from build123d import *

# Parameters (mm, degrees)
BOSS_EXTRUDE2_DEPTH = 20
SKETCH3_R           = 30
SKETCH3_R_2         = 15
BOSS_EXTRUDE3_DEPTH = 30
SKETCH5_R           = 15
BOSS_EXTRUDE4_DEPTH = 70
FILLET1_R           = 5


with BuildPart() as part:
    # Sketch1 → Boss-Extrude2 (new body)
    with BuildSketch(Plane(origin=(0, 0, 0), x_dir=(1, 0, 0), z_dir=(0, 1, 0))):
        with BuildLine():
            Line((-121.213203436, 21.213203436), (-21.213203436, 121.213203436))
            ThreePointArc((-21.213203436, 121.213203436), (0, 70), (21.213203436, 121.213203436))
            Line((21.213203436, 121.213203436), (121.213203436, 21.213203436))
            ThreePointArc((121.213203436, 21.213203436), (72.283614025, 11.480502971), (100, -30))
            Line((100, -30), (-100, -30))
            ThreePointArc((-100, -30), (-72.283614025, 11.480502971), (-121.213203436, 21.213203436))
        make_face()
    extrude(amount=BOSS_EXTRUDE2_DEPTH)

    # Sketch3 → Boss-Extrude3 (add)
    # profile 1 of 3: a face of its own
    with BuildSketch(Plane.XZ):
        with Locations(Location((0, -100, 0), (0, 0, 270))):
            Circle(SKETCH3_R)
        with Locations(Location((0, -100, 0), (0, 0, 270))):
            Circle(SKETCH3_R_2, mode=Mode.SUBTRACT)
    # profile 2 of 3: a face of its own
    with BuildSketch(Plane.XZ):
        with Locations(Location((100, 0, 0), (0, 0, 270))):
            Circle(SKETCH3_R)
        with Locations(Location((100, 0, 0), (0, 0, 270))):
            Circle(SKETCH3_R_2, mode=Mode.SUBTRACT)
    # profile 3 of 3: a face of its own
    with BuildSketch(Plane.XZ):
        with Locations(Location((-100, 0, 0), (0, 0, 270))):
            Circle(SKETCH3_R)
        with Locations(Location((-100, 0, 0), (0, 0, 270))):
            Circle(SKETCH3_R_2, mode=Mode.SUBTRACT)
    extrude(amount=-BOSS_EXTRUDE3_DEPTH)

    # Sketch5 → Boss-Extrude4 (add)
    with BuildSketch(Plane.XY.offset(30)):
        with BuildLine():
            Line((-20, 49.8), (-20, 0))
            Line((-20, 0), (20, 0))
            Line((20, 0), (20, 49.8))
            ThreePointArc((20, 49.8), (0, 69.8), (-20, 49.8))
        make_face()
        with Locations((0, 49.8)):
            Circle(SKETCH5_R, mode=Mode.SUBTRACT)
    extrude(amount=-BOSS_EXTRUDE4_DEPTH)

    # Fillet1
    fillet1_edges = [part.edges().sort_by_distance(p)[0] for p in [
        (20, 20, -5),
        (-20, 20, -5),
    ]]
    fillet(fillet1_edges, radius=FILLET1_R)


solid = part.part
The listing builds one solid part. Answer for the finished solid, in the listing's coordinates (mm). A direction names the side the tool comes from. Give positions to 0.01 mm unless a question says otherwise; leave off trailing zeros. Write each loop counter-clockwise with the first axis right and the second up, starting at its lowest first coordinate (ties: lowest second). Pieces come first, ordered by that corner, then holes.
1) Given P1, Ø24, axis at x = 0, y = 49.8, coming from the -Z side; P2, Ø1.5, axis at x = -66.5, z = 10, coming from the +Y side; P3, Ø12, axis at y = 10, z = -21, coming from the -X side; P4, Ø12, axis at y = 45.5, z = -3, coming from the +X side, each flat-ended and moving along its own axis, determine where each tip first touches the part or whether it passes through.
2) Section D-D (y = 7) is taken. Write down the section's boundary in (x, z), and give its area (3 significant figures).
3) Find the intervals of material crossed by L1, parallel to X at y = 11, z = 0; L2, parallel to Y at x = 0, z = -12.5; L3, parallel to X at y = 18, z = 9, in increasing order.
4) Section C-C (x = 92) is taken. Write down the section's boundary in (y, z).
5) Section A-A (x = 0) is taken. Write down the section's boundary in (y, z), and give its area (3 significant figures).
6) For a pull along X with two mould halves and no side action, classify faces 4 (the face through (0.44, 69.795, -4.51)), 5 (the face through (20, 37, -5)), 6 (the face through (0, 20, 30)) as pulls with the +X half, pulls with the -X half, needs draft (parallel to the pull), parting line crosses it, or undercut.
7) A tool of negligible diameter and unlimited length cuts with its end or side. For faces 1 (the face through (0, 34, -40)), 2 (the face through (129.745, 18.123, 3.905)), 3 (the face through (114, 30, -6)), from which of +Z, -Z, +X, -X, +Y, -Y can it reach the whole face along a straight path? Write none if from no direction.
8) Section B-B (z = 11.5) is taken. Write down the section's boundary in (x, y).
Response:
1. P1: passes through
1. P2: stops at y = 20
1. P3: stops at x = -125.98
1. P4: stops at x = 20
2. outline: (-121.21, -21.21) - (-21.21, -121.21) arc R30 ccw to (21.21, -121.21) - (121.21, -21.21) arc R30 ccw to (100, 30) - (-100, 30) arc R30 ccw to start; hole circle Ø30 at (-100, 0); hole circle Ø30 at (0, -100); hole circle Ø30 at (100, 0)
2. area: 25,200 mm2
3. L1: x = -130 to -115, -85 to 85, 115 to 130
3. L2: y = 0 to 34.8, 64.8 to 69.8
3. L3: x = -128.62 to -112, -88 to 88, 112 to 128.62
4. outline: (0, -50.43) - (20, -50.43) - (20, -28.91) - (30, -28.91) - (30, -12.69) - (0, -12.69) - close; (0, 12.69) - (30, 12.69) - (30, 28.91) - (20, 28.91) - (20, 30) - (0, 30) - close
5. outline: (0, -130) - (30, -130) - (30, -115) - (0, -115) - close; (0, -85) - (30, -85) - (30, -70) - (20, -70) - (20, -40) - (34.8, -40) - (34.8, 30) - (0, 30) - close; (64.8, -40) - (69.8, -40) - (69.8, 30) - (64.8, 30) - close
5. area: 4,290 mm2
6. face 4: parting line crosses it
6. face 5: undercut
6. face 6: needs draft
7. face 1: +X, -X, +Y
7. face 2: +Y
7. face 3: +Z, -Z, +X, +Y
8. outline: (-127.71, 0) - (-109.63, 0) - (-109.63, 30) - (-127.71, 30) - close; (-90.37, 0) - (90.37, 0) - (90.37, 30) - (72.29, 30) - (72.29, 20) - (25, 20) arc R5 cw to (20, 25) - (20, 49.8) arc R20 ccw to (-20, 49.8) - (-20, 25) arc R5 cw to (-25, 20) - (-72.29, 20) - (-72.29, 30) - (-90.37, 30) - close; (109.63, 0) - (127.71, 0) - (127.71, 30) - (109.63, 30) - close; hole circle Ø30 at (0, 49.8)
